Geometry: final body of the model. Coordinates: model frame, mm. A direction names the side the tool comes from. Give positions to 0.01 mm unless a question says otherwise; leave off trailing zeros. Loops run counter-clockwise (first coordinate to the right, second up) from the corner with the lowest first, then second, coordinate; pieces in that order, holes last. Notation, with made-up numbers: (-34, -23) - (-24, -23) arc R12 ccw to (-24, -16) - close; hole circle Ø9 at (39, -8.5). An arc over 180 degrees is marked (long way). Answer in a Markdown table with one row per item.
Autodesk Inventor part; units mm, degrees
ref_plane "Work Plane1" through (0, 0, 27.94) normal (0, 0, 1) x (1, 0, 0)
ref_plane "YZ Plane" through (0, 0, 0) normal (1, 0, 0) x (0, 1, 0)
ref_plane "XZ Plane" through (0, 0, 0) normal (0, 1, 0) x (-1, 0, 0)
sketch "Sketch1" plane through (0, 0, 0) normal (0, 0, 1) x (1, 0, 0)
  line L0 (0, 0) -> (3.302, 0)
  line L1 (3.302, 0) -> (3.302, -27.94)
  line L2 (3.302, -27.94) -> (0, -27.94)
  line L3 (0, -27.94) -> (0, 0)
  dimension "d0" = 3.302
  dimension "d1" = 27.94
extrude "Extrusion1" add sketch "Sketch1" along normal blind 2.54
sketch "Sketch2" plane through (0, 0, 2.54) normal (0, 0, 1) x (1, 0, 0)
  line L0 (3.302, 0) -> (0, 0)
  line L1 (0, 0) -> (0, -27.94)
  line L2 (0, -27.94) -> (3.302, -27.94)
  line L3 (3.302, -27.94) -> (3.302, 0)
ref_plane "Work Plane1" through (0, 0, 27.94) normal (0, 0, 1) x (1, 0, 0)
sketch "Sketch3" plane through (0, 0, 27.94) normal (0, 0, 1) x (1, 0, 0)
  line L0 (0, -6.985) -> (3.302, -6.985)
  line L1 (3.302, -6.985) -> (3.302, -20.955)
  line L2 (3.302, -20.955) -> (0, -20.955)
  line L3 (0, -20.955) -> (0, -6.985)
  line L4 (0, -27.94) -> (3.302, -27.94)
  line L5 (0, 0) -> (0, -27.94)
  dimension "d5" = 3.302
  dimension "d6" = 13.97
  dimension "d7" = 6.985
  dimension "d8" = 0
loft "Loft1" add profiles "Sketch2", "Sketch3"
sketch "Sketch4" plane through (3.302, -27.94, 0) normal (1, 0, 0) x (0, 0, -1)
  line L0 (0, 0) -> (0, 27.94)
  line L1 (-2.54, 0) -> (-27.94, 6.985)
  line L2 (0, 27.94) -> (-2.54, 27.94)
  line L3 (-2.54, 27.94) -> (-2.54, 0)
  line L4 (-2.54, 0) -> (0, 0)
  line L5 (0, 0) -> (0, 27.94)
  line L6 (-2.54, 27.94) -> (-27.94, 20.955)
  line L7 (-27.94, 20.955) -> (-2.54, 20.955)
  line L8 (-2.54, 20.955) -> (-2.54, 18.415)
  line L9 (-2.54, 18.415) -> (-27.94, 18.415)
  line L10 (-27.94, 18.415) -> (-27.94, 20.955)
  line L11 (-27.94, 6.985) -> (-2.54, 6.985)
  line L12 (-2.54, 6.985) -> (-2.54, 9.525)
  line L13 (-2.54, 9.525) -> (-27.94, 9.525)
  line L14 (-27.94, 9.525) -> (-27.94, 6.985)
  dimension "d13" = 2.54
  dimension "d14" = 2.54
extrude "Extrusion2" add sketch "Sketch4" along normal blind 8.89 contours L4 L3 L2 L0 | L1 L11 L3 | L14 L13 L3 L11 | L3 L9 L10 L7
sketch "Sketch5" plane through (12.192, -27.94, 0) normal (1, 0, 0) x (0, 0, -1)
  line L0 (-27.94, 20.955) -> (-27.94, 6.985)
  line L1 (-27.94, 6.985) -> (-2.54, 6.985)
  line L2 (0, 0) -> (-2.54, 0)
  line L3 (-2.54, 0) -> (-2.54, 6.985)
  line L4 (-2.54, 0) -> (-27.94, 6.985)
  line L5 (-2.54, 0) -> (-27.94, 6.985)
  point P0 (0, 27.94)
extrude "Extrusion3" cut sketch "Sketch5" against normal blind 8.89
sketch "Sketch6" plane through (12.192, -20.955, 2.54) normal (0, -1, 0) x (1, 0, 0)
  line L0 (-2.286, 5.08) -> (-4.445, 5.08)
  line L1 (-4.445, 5.08) -> (-4.445, 0)
  line L2 (-4.445, 0) -> (-2.286, 0)
  line L3 (-2.286, 0) -> (-2.286, 5.08)
  line L4 (-8.89, 0) -> (0, 0)
  line L5 (0, 25.4) -> (0, 0)
  point P0 (-12.192, -2.54)
  dimension "d19" = 0
  dimension "d20" = 5.08
  dimension "d21" = 2.286
  dimension "d22" = 2.159
extrude "Extrusion4" cut sketch "Sketch6" against normal blind 25.4
sketch "Sketch7" plane through (12.192, -20.955, 2.54) normal (0, -1, 0) x (1, 0, 0)
  line L0 (0, 14.9225) -> (-0.635, 14.9225)
  line L1 (-0.635, 14.9225) -> (-0.635, 10.4775)
  line L2 (-0.635, 10.4775) -> (0, 10.4775)
  line L3 (0, 10.4775) -> (0, 14.9225)
  line L4 (0, 25.4) -> (0, 0)
  line L5 (-8.89, 25.4) -> (0, 25.4)
  point P0 (-12.192, -2.54)
  dimension "d25" = 0.635
  dimension "d26" = 4.445
  dimension "d27" = 0
  dimension "d28" = 10.4775
extrude "Extrusion5" cut sketch "Sketch7" against normal blind 25.4
sketch "Sketch8" plane through (12.192, -27.94, 0) normal (1, 0, 0) x (0, 0, -1)
  line L0 (-2.54, 18.415) -> (-2.54, 20.955)
  line L1 (-13.0175, 20.955) -> (-13.0175, 18.415)
  line L2 (-2.54, 20.955) -> (-13.0175, 20.955)
  line L3 (-13.0175, 20.955) -> (-13.0175, 18.415)
  line L4 (-13.0175, 18.415) -> (-2.54, 18.415)
  line L5 (-2.54, 18.415) -> (-2.54, 20.955)
  line L6 (-2.54, 9.525) -> (-13.0175, 9.525)
  line L7 (-27.94, 6.985) -> (-2.54, 6.985)
  line L8 (-2.54, 9.525) -> (-13.0175, 9.525)
  line L9 (-13.0175, 9.525) -> (-13.0175, 6.985)
  line L10 (-13.0175, 6.985) -> (-2.54, 6.985)
  line L11 (-2.54, 6.985) -> (-2.54, 9.525)
  line L12 (-17.4625, 20.955) -> (-13.0175, 20.955)
  line L13 (-27.94, 9.525) -> (-27.94, 18.415)
  line L14 (-17.4625, 20.955) -> (-27.94, 20.955)
  line L15 (-27.94, 20.955) -> (-27.94, 18.415)
  line L16 (-27.94, 18.415) -> (-17.4625, 18.415)
  line L17 (-17.4625, 18.415) -> (-17.4625, 20.955)
  line L18 (-17.4625, 6.985) -> (-17.4625, 9.525)
  line L19 (-17.4625, 9.525) -> (-27.94, 9.525)
  line L20 (-27.94, 9.525) -> (-27.94, 6.985)
  line L21 (-27.94, 6.985) -> (-17.4625, 6.985)
  line L22 (-17.4625, 6.985) -> (-17.4625, 9.525)
  point P0 (0, 27.94)
extrude "Extrusion6" add sketch "Sketch8" along normal blind 3.81
sketch "Sketch9" plane through (0, 0, 0) normal (0, 0, -1) x (-1, 0, 0)
  point P0 (0, 0)
sketch "Sketch10" plane through (0, 0, 0) normal (0, 0, -1) x (-1, 0, 0)
  line L0 (-12.192, -27.94) -> (0, -27.94)
  line L1 (0, -27.94) -> (0, 0)
  line L2 (-12.192, -27.94) -> (0, -27.94)
  line L3 (0, -27.94) -> (0, 0)
  line L4 (0, 0) -> (-12.192, 0)
  line L5 (-12.192, 0) -> (-12.192, -27.94)
extrude "Extrusion7" add sketch "Sketch10" along normal blind 6.35
sketch "Sketch13" plane through (12.192, -27.94, 0) normal (1, 0, 0) x (0, 0, -1)
  point P0 (0, 27.94)
sketch "Sketch14" plane through (12.192, -27.94, 0) normal (1, 0, 0) x (0, 0, -1)
  point P0 (0, 27.94)
sketch "Sketch15" plane through (12.192, -27.94, 0) normal (1, 0, 0) x (0, 0, -1)
  circle A0 centre (1.905, 13.97) radius 2.54
  line L0 (6.35, 27.94) -> (6.35, 0)
  line L1 (-2.54, 27.94) -> (6.35, 27.94)
  point P0 (0, 27.94)
  dimension "d41" = 5.08
  dimension "d42" = 4.445
  dimension "d43" = 13.97
extrude "Extrusion9" cut sketch "Sketch15" against normal blind 254
sketch "Sketch17" plane through (12.192, -27.94, 0) normal (1, 0, 0) x (0, 0, -1)
  circle A0 centre (1.905, 13.97) radius 2.54
  circle A1 centre (1.905, 13.97) radius 2.54
  point P0 (0, 27.94)
extrude "Extrusion10" add sketch "Sketch17" against normal blind 12.192
properties part number "Talon for encoder"
Q1. Cut plane D-D (x = 10.5). Output: boundary loops of the cut face in (y, z) (3 decimals), and give its area (3 significant figures).
Check values:
| item | result |
|---|---|
| outline | (-27.94, -6.35) - (0, -6.35) - (0, 2.54) - (-6.985, 2.54) - (-6.985, 27.94) - (-9.525, 27.94) - (-9.525, 2.54) - (-18.415, 2.54) - (-18.415, 27.94) - (-20.955, 27.94) - (-20.955, 2.54) - (-27.94, 2.54) - close |
| area | 377 mm² |
Q2. First-contact query: pin 1 (6.5 mm diameter, centred on x = 9.5, z = 21, fed in from -Y) (3 decimals); pin 2 (2.5 mm diameter, centred on y = -13, z = 0, fed in from +X); pin 3 (4 mm diameter, centred on x = 10, z = 11, fed in from +Y) (3 decimals); pin 4 (1.5 mm diameter, centred on x = 14, y = -12.5, fed in from -Z). Flat tips, straight axial feed; report the tip coordinate or a pass-through.
Check values:
| item | result |
|---|---|
| pin 1 | y = -20.955 |
| pin 2 | x = 12.19 |
| pin 3 | y = -6.985 |
| pin 4 | through |
Q3. Draft query along Y for faces 1 (the flat face through (3.302, -14, 15)), 2 (the flat face through (10, -20.955, 15)), 3 (the flat face through (14, -8, 2.54)), 4 (the flat face through (10, -18.415, 15)). Return one class per face: pulls with the +Y half, pulls with the -Y half, needs draft (parallel to the pull), parting line crosses it, or undercut.
Check values:
| item | result |
|---|---|
| face 1 | undercut |
| face 2 | pulls with the -Y half |
| face 3 | needs draft |
| face 4 | undercut |
Q4. Cut plane C-C (y = -19). Output: boundary loops of the cut face in (x, z).
Check values:
| item | result |
|---|---|
| outline | (0, -6.35) - (12.19, -6.35) - (12.19, 2.54) - (16, 2.54) - (16, 13.02) - (11.56, 13.02) - (11.56, 17.46) - (16, 17.46) - (16, 27.94) - (0, 27.94) - close; hole (7.75, 2.54) - (9.91, 2.54) - (9.91, 7.62) - (7.75, 7.62) - close |
Q5. Cut plane A-A (x = 14.5). Output: boundary loops of the cut face in (y, z) (1 decimal).
Check values:
| item | result |
|---|---|
| outline | (-21, 2.5) - (-18.4, 2.5) - (-18.4, 13) - (-21, 13) - close; (-21, 17.5) - (-18.4, 17.5) - (-18.4, 27.9) - (-21, 27.9) - close; (-9.5, 2.5) - (-7, 2.5) - (-7, 13) - (-9.5, 13) - close; (-9.5, 17.5) - (-7, 17.5) - (-7, 27.9) - (-9.5, 27.9) - close |
Q6. Material intervals for line 1 along Y through (x, z) = (13.75, 24) (3 decimals); line 2 along Z through (x, y) = (9.25, -9.25); line 3 along Z through (x, y) = (5, -14), sorted ascending.
Check values:
| item | result |
|---|---|
| line 1 | -20.955 to -18.415, -9.525 to -6.985 |
| line 2 | -6.35 to 2.54, 7.62 to 27.94 |
| line 3 | -6.35 to 2.54 |
Q7. Reachability of faces 5 (the flat face through (11.557, -20, 15)), 6 (the flat face through (3.302, -5, 9)), 7 (the flat face through (7.747, -20, 5)), 8 (the flat face through (14, -20, 2.54)) from +Z, -Z, +X, -X, +Y, -Y: full face, straight path, thin tool, end or side. Return the list, or none.
Check values:
| item | result |
|---|---|
| face 5 | +X, +Y, -Y |
| face 6 | +Z, +X, +Y |
| face 7 | +Y, -Y |
| face 8 | -Z, +X, +Y, -Y |
Q8. Cut plane B-B (z = 6). Output: boundary loops of the cut face in (x, y) (1 decimal).
Check values:
| item | result |
|---|---|
| outline | (0, -27) - (3.3, -27) - (3.3, -21) - (7.7, -21) - (7.7, -18.4) - (3.3, -18.4) - (3.3, -9.5) - (7.7, -9.5) - (7.7, -7) - (3.3, -7) - (3.3, -1) - (0, -1) - close; (9.9, -21) - (16, -21) - (16, -18.4) - (9.9, -18.4) - close; (9.9, -9.5) - (16, -9.5) - (16, -7) - (9.9, -7) - close |
